The listing builds one solid part. Answer for the finished solid, in the listing's coordinates (mm). Face numbers are marked on the shaded views. A direction names the side the tool comes from. Round coordinates to 2 decimals unless told otherwise and drop trailing zeros. Write each loop counter-clockwise with the first axis right and the second up, starting at its lowest first coordinate (ties: lowest second). Pieces come first, ordered by that corner, then holes.
Item 1: Find section A-A on z = -6. Give the vertices of the cut face in (x, y), then the cut area to 3 significant figures.
Item 2: Find the intervals of material crossed by probe 1 along X at (y, z) = (-12.5, -21); probe 2 along Z at (x, y) = (-17, 15); probe 3 along Y at (x, z) = (18.5, -22.5), in increasing order.
Item 3: Find section B-B on z = 14. Give the vertices of the cut face in (x, y), then the cut area to 3 significant figures.
Item 4: A tool of negligible diameter and unlimited length cuts with its end or side. For the marked faces 5, 6 and 7, from which of +Z, -Z, +X, -X, +Y, -Y can it reach the whole face along a straight path? Write none if from no direction.
Item 5: Each of these flat-tipped pins is pushed along its axis until it touches: pin 1 (3 mm diameter, centred on y = -7, z = -22, fed in from +X); pin 2 (6 mm diameter, centred on x = 15, z = -12, fed in from +Y); pin 3 (12 mm diameter, centred on y = 3.5, z = -1, fed in from -X); pin 4 (5 mm diameter, centred on y = 4.5, z = 13.5, fed in from +X). Where does it stop, or does it pass through?
Item 6: For a pull along Z with two mould halves and no side action, classify the marked faces 1, 2, 3 and 4 as +Z half, -Z half, draft (parallel to the pull), parting line (faces both ways), or undercut.
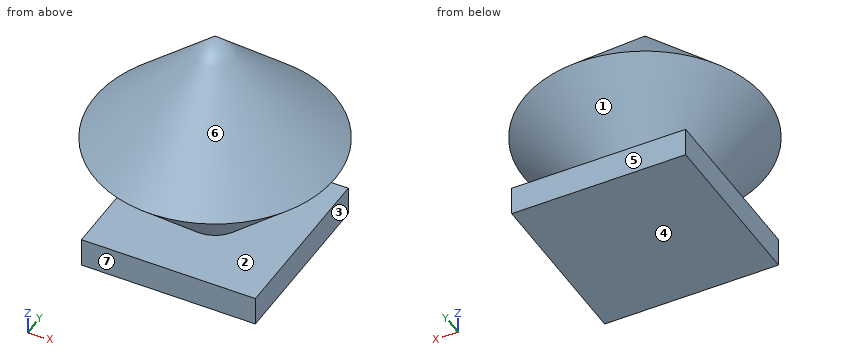
```python
from build123d import *

# Parameters (mm, degrees)
F3_DEPTH      = 19.05
F3_DEPTH_BACK = 19.05


with BuildPart() as f1:
    # F0 (on Front) → F1 (revolve)
    with BuildSketch(Plane.XZ):
        Polygon((26.343262, 0), (0, 25.4), (0, -25.4), align=None)
    revolve(axis=Axis((0, 0, 0), (0, 0, -1)))

    # F2 (on Right) → F3 (join, two sides)
    with BuildSketch(Plane.YZ) as f3_sk:
        Polygon((-19.143354, -25.375442), (-0.093354, -25.375442), (18.956646, -25.375442), (18.956646, -19.025442), (-0.093354, -19.025442), (-19.143354, -19.025442), align=None)
    extrude(amount=F3_DEPTH)
    extrude(f3_sk.sketch, amount=-F3_DEPTH_BACK)


solid = f1.part
```
Check values:
1. outline: circle Ø40.24 at (0, 0)
1. area: 1,270 mm2
2. probe 1: x = -19.05 to 19.05
2. probe 2: z = -25.38 to -19.03, -3.54 to 3.54
2. probe 3: y = -19.14 to 18.96
3. outline: circle Ø23.65 at (0, 0)
3. area: 439 mm2
4. face 5: -Z, +X, -X, +Y
4. face 6: +Z
4. face 7: -Z, +X, -X, -Y
5. pin 1: stops at x = 19.05
5. pin 2: stops at y = 9.71
5. pin 3: stops at x = -26.34
5. pin 4: stops at x = 14.34
6. face 1: undercut
6. face 2: undercut
6. face 3: draft
6. face 4: -Z half
